Input: part model. Units: mm. Frame: model coordinates. Coordinates: 2 decimals unless noted, no trailing zeros. Loops run counter-clockwise (first coordinate to the right, second up) from the corner with the lowest first, then second, coordinate; pieces in that order, holes last. Notation, with made-up numbers: (54, 78) - (89, 78) arc R26 ccw to (89, 103) - close; hole circle Ø1 at (-28.75, 24). An arc over 180 degrees is marked (long way). Use a Markdown table: item, result. Add a question column.
1. Ray query, L1, parallel to Z at x = -298.5, y = 166.5; L2, parallel to X at y = 129.5, z = 146; L3, parallel to X at y = 52.5, z = 84.5. Return the intervals inside material, ascending. Write a range as [from, to].
2. Section query D-D on z = 24.5. Return the cut outline in (x, y), then the cut area to 3 significant figures.
3. Draft query along Z for faces 1 (the face through (-310, -97.6, 142.4)), 2 (the face through (-310, -97.6, 92.5)), 3 (the face through (-4, -4, 180)). Return one class per face: released by +Z, released by -Z, zero draft, split by the parting line, or undercut.
4. Section query A-A on y = 0. Return the cut outline in (x, z).
5. Section query C-C on z = 159. Return the cut outline in (x, y), then the cut area to 3 significant figures.
6. Contact query for flat-ended pins moving along their axis: P1, Ø1, axis at x = 244.5, y = 223.5, coming from the +Z side; P2, Ø4, axis at x = 46.5, z = 74.5, coming from the -Y side; P3, Ø4, axis at x = 9, z = 129.5, coming from the -Y side. Output: stop coordinate, or through.
```python
from build123d import *


with BuildPart() as f1:
    # F0 (on Front) → F1 (revolve)
    with BuildSketch(Plane.XZ):
        with BuildLine():
            Line((-325, 0), (0, 0))
            Line((0, 0), (0, 180))
            Line((0, 180), (-295, 180))
            ThreePointArc((-295, 180), (-303.786797, 158.786797), (-325, 150))
            Line((-325, 150), (-325, 135))
            ThreePointArc((-325, 135), (-345, 115), (-325, 95))
            Line((-325, 95), (-325, 90))
            ThreePointArc((-325, 90), (-370, 45), (-325, 0))
        make_face()
    revolve(axis=Axis((0, 0, 90), (0, 0, 1)))


solid = f1.part
```
Resolved:
| question | item | result |
|---|---|---|
| 1 | L1 | [3.25, 86.75], [104.14, 125.86] |
| 1 | L2 | [-298.09, 298.09] |
| 1 | L3 | [-342.56, 342.56] |
| 2 | outline | circle Ø730.12 at (0, 0) |
| 2 | area | 419,000 mm² |
| 3 | face 1 | zero draft |
| 3 | face 2 | undercut |
| 3 | face 3 | released by +Z |
| 4 | outline | (-325, 0) - (325, 0) arc R45 ccw to (325, 90) - (325, 95) arc R20 ccw to (325, 135) - (325, 150) arc R30 cw to (295, 180) - (-295, 180) arc R30 cw to (-325, 150) - (-325, 135) arc R20 ccw to (-325, 95) - (-325, 90) arc R45 ccw to start |
| 5 | outline | circle Ø607.15 at (0, 0) |
| 5 | area | 290,000 mm² |
| 6 | P1 | z = 134.15 |
| 6 | P2 | y = -357.63 |
| 6 | P3 | y = -340.49 |
